Geometry: final body of the model. Coordinates: model frame, mm. Give positions to 0.01 mm unless a question says otherwise; leave off trailing zeros. Order: outer loops, then holes, each group sorted by start corner. A loop starts at its lowest first (then second) coordinate and runs counter-clockwise, first axis right, second up. Notation, with made-up numbers: M 32.25,39.25 L 62.25,39.25 A23 cw 62.25,58.25 Z; hole C 19.5,78.5 d4. An arc over 180 degrees is marked long. Use CSV: the item, a comma, the result in double quotes.
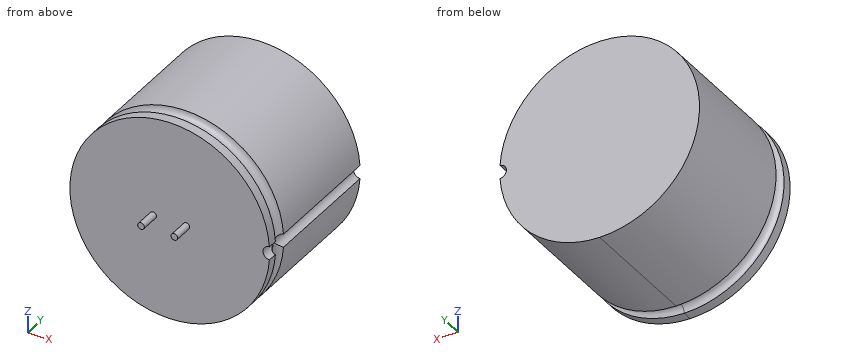
```python
from build123d import *

# Parameters (mm, degrees)
SKETCH_2_R          = 30
EXTRUDE_1_DEPTH     = 45
SKETCH_3_R          = 2
SKETCH_4_R          = 1
EXTRUDE_2_DEPTH     = 6
SKETCH_5_R          = 2
CUT_EXTRUDE_1_DEPTH = 45


with BuildPart() as part:
    # Эскиз2 → Бобышка-Вытянуть1 (new body)
    with BuildSketch(Plane(origin=(0, 0, 0), x_dir=(1, 0, 0), z_dir=(0, 1, 0))):
        with Locations(Location((0, 0, 0), (0, 0, 90))):
            Circle(SKETCH_2_R)
    extrude(amount=EXTRUDE_1_DEPTH)

    # Эскиз3 → Вырез-Повернуть1 (revolve, cut)
    with BuildSketch(Plane(origin=(0, 0, 0), x_dir=(0, 0, -1), z_dir=(1, 0, 0)), mode=Mode.PRIVATE) as cut_revolve_1_sk:
        with Locations((-30, 5)):
            Circle(SKETCH_3_R)
    revolve(cut_revolve_1_sk.sketch.rotate(Axis((0, 0, 0), (0, 1, 0)), 180), axis=Axis((0, 0, 0), (0, 1, 0)), mode=Mode.SUBTRACT)

    # Эскиз4 → Бобышка-Вытянуть2 (add)
    with BuildSketch(Plane.XZ):
        with Locations(Location((5, 0, 0), (0, 0, 90))):
            Circle(SKETCH_4_R)
        with Locations(Location((-5, 0, 0), (0, 0, 90))):
            Circle(SKETCH_4_R)
    extrude(amount=EXTRUDE_2_DEPTH)

    # Эскиз5 → Вырез-Вытянуть1 (cut)
    with BuildSketch(Plane.XZ):
        with Locations((30, 0)):
            Circle(SKETCH_5_R)
    extrude(amount=-CUT_EXTRUDE_1_DEPTH, mode=Mode.SUBTRACT)


solid = part.part
```
1. Section A-A, the plane y = 31. Return the cut outline in (x, z).
Answer:
outline,"M 29.93,-2 A2 cw 29.93,2 A30 ccw long Z"
2. Line query: line 1 (Y direction, x = 24, z = 8); line 2 (Y direction, x = -27, z = -11); line 3 (X direction, y = 17, z = -20). Output: solid intervals per line, ascending.
Answer:
line 1,"0 to 45"
line 2,"0 to 3.19, 6.81 to 45"
line 3,"-22.36 to 22.36"
3. Pin query (flat end, axial travel): pin 1 Ø1 at (x, y) = (-12, 12.5) entering from -Z; pin 2 Ø1 at (y, z) = (14.5, -16) entering from -X; pin 3 Ø4 at (x, y) = (6.5, 11.5) entering from -Z. Return the tip coordinate at first contact, or that it passes through.
Answer:
pin 1,"z = -27.71"
pin 2,"x = -25.69"
pin 3,"z = -29.66"
